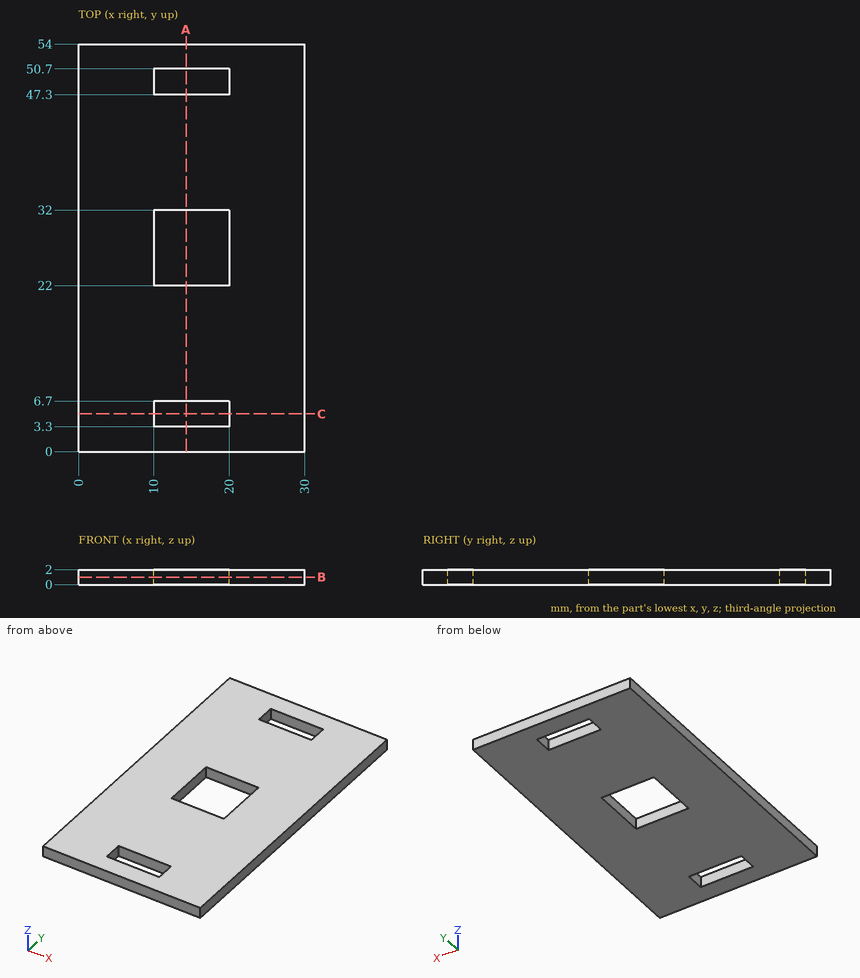
Geometry: see drawing. Coordinates: mm, zero at the bounding-box minimum. Give positions to 0.01 mm unless a question says otherwise; leave off trailing zeros. Order: outer loops, then holes, each group sorted by start corner. A loop starts at its lowest first (then second) coordinate and runs counter-clockwise, first axis right, second up. Notation, with made-up numbers: (-19, 60.25) -> (4, 60.25) arc R23 ccw to (4, 73.25) -> close; hole circle Ø4 at (66, 68). An arc over 180 degrees is marked (long way). Write each question's results on one line, items separated by ' | '. Start each with the question number.
1) Line query: line 1 (Y direction, x = 16.5, z = 0.65); line 2 (X direction, y = 27, z = 1.7). Output: solid intervals per line, ascending. Write a range as from..to.
2) First-contact query: pin 1 (1 mm diameter, centred on y = 33.5, z = 1.5, fed in from -X). Flat tip, straight axial feed; report the tip coordinate or a pass-through.
3) Section B-B (z = 1). Return loops of the section in (x, y).
4) Section A-A (x = 14.25). Return loops of the section in (y, z).
5) Section C-C (y = 5). Return loops of the section in (x, z).
Calculated:
1) line 1: 0..3.3, 6.7..22, 32..47.3, 50.7..54 | line 2: 0..10, 20..30
2) pin 1: x = 0
3) outline: (0, 0) -> (30, 0) -> (30, 54) -> (0, 54) -> close; hole (10, 3.3) -> (20, 3.3) -> (20, 6.7) -> (10, 6.7) -> close; hole (10, 22) -> (20, 22) -> (20, 32) -> (10, 32) -> close; hole (10, 47.3) -> (20, 47.3) -> (20, 50.7) -> (10, 50.7) -> close
4) outline: (0, 0) -> (3.3, 0) -> (3.3, 2) -> (0, 2) -> close; (6.7, 0) -> (22, 0) -> (22, 2) -> (6.7, 2) -> close; (32, 0) -> (47.3, 0) -> (47.3, 2) -> (32, 2) -> close; (50.7, 0) -> (54, 0) -> (54, 2) -> (50.7, 2) -> close
5) outline: (0, 0) -> (10, 0) -> (10, 2) -> (0, 2) -> close; (20, 0) -> (30, 0) -> (30, 2) -> (20, 2) -> close
